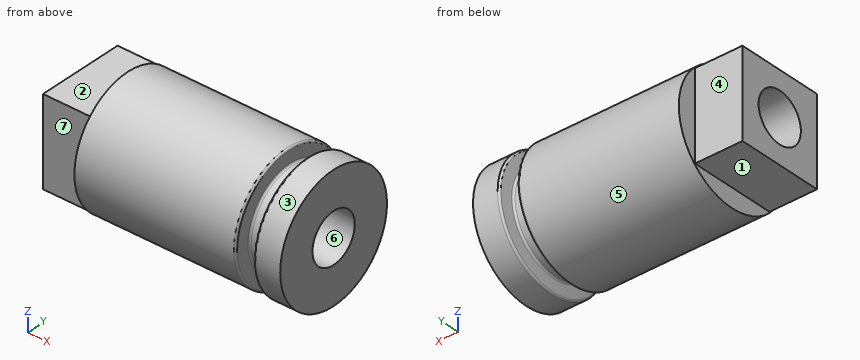
from build123d import *

# Parameters (mm, degrees)
F2_W     = 17.4498
F2_H     = 17.4498
F3_DEPTH = 9.525
F4_R     = 4.953
F5_DEPTH = 50.801


with BuildPart() as f1:
    # F0 (on Front) → F1 (revolve)
    with BuildSketch(Plane.XZ):
        with BuildLine():
            Line((11.316179, 12.4968), (-20.6375, 12.4968))
            Line((-20.6375, 12.4968), (-20.6375, 0))
            Line((-20.6375, 0), (20.6375, 0))
            Line((20.6375, 0), (20.6375, 12.4968))
            Line((20.6375, 12.4968), (15.709421, 12.4968))
            ThreePointArc((15.709421, 12.4968), (15.452021, 12.396703), (15.329871, 12.149006))
            Line((15.329871, 12.149006), (15.130728, 9.872794))
            ThreePointArc((15.130728, 9.872794), (15.008578, 9.625097), (14.751178, 9.525))
            Line((14.751178, 9.525), (12.274422, 9.525))
            ThreePointArc((12.274422, 9.525), (12.017022, 9.625097), (11.894872, 9.872794))
            Line((11.894872, 9.872794), (11.695729, 12.149006))
            ThreePointArc((11.695729, 12.149006), (11.573579, 12.396703), (11.316179, 12.4968))
        make_face()
    revolve(axis=Axis((-2.210241, 0, 0), (-1, 0, 0)))

    # F2 (on face) → F3 (join)
    with BuildSketch(Plane(origin=(-20.6375, 0, 0), x_dir=(0, -1, 0), z_dir=(-1, 0, 0))):
        Rectangle(F2_W, F2_H)
    extrude(amount=F3_DEPTH)

    # F4 (on face) → F5 (cut, through all)
    with BuildSketch(Plane.YZ.offset(20.6375)):
        Circle(F4_R)
    extrude(amount=-F5_DEPTH, mode=Mode.SUBTRACT)


solid = f1.part
For this review, take the finished solid that the model builds, in its own axes (mm). Face numbers are marked on the shaded views. A direction names the side the tool comes from. Give positions to 0.01 mm unless a question says otherwise; leave off trailing zeros. Order: outer loops, then holes, each group sorted by start corner. A loop starts at its lowest first (then second) coordinate and runs counter-clockwise, first axis right, second up. Notation, with made-up numbers: (63, 17) - (84, 17) arc R10 ccw to (84, 34) - close; hole circle Ø2 at (42, -11). An arc over 180 degrees is marked (long way). Answer as a JSON object with one key per item and string values. Group by question number.
Item 1: Machinability: for the marked faces 1, 2, 3 and 4, which of the approach directions +Z, -Z, +X, -X, +Y, -Y give a long, thin tool a straight path to every point of the face, cutting with its end or side? Answer none if there is none.
Item 2: Draft analysis for pull direction Z (two halves, no side actions). For the marked faces 5, 6 and 7, state which applies: pulls with the +Z half, pulls with the -Z half, needs draft (parallel to the pull), parting line crosses it, or undercut.
Item 3: Clearance check with flat-ended pins moving along their axes: pin 1 Ø1.5 at (x, y) = (-11.5, -7) entering from -Z; pin 2 Ø5 at (x, z) = (-25, 0) entering from -Y; pin 3 Ø5 at (x, y) = (-3, 7) entering from -Z. State where each tip first meets the part, or that it passes through.
Item 4: Take a section at A-A on z = 0. Give the boundary of the cut face in (x, y) (1 decimal), and give its area (3 significant figures).
Item 5: Take a section at D-D on x = -9. Give the boundary of the cut face in (y, z).
Item 6: Take a section at C-C on x = -25.5. Give the boundary of the cut face in (y, z), and give its area (3 significant figures).
Item 7: Wall thickness on line 1 along X through (y, z) = (10.5, 6) (1 decimal); line 2 along Z through (x, y) = (-18, 2.5); line 3 along Z through (x, y) = (-1.5, 4.25): over which ranges is each line inside the solid? List them lowest first.
Reported:
{
 "1": {"face 1": "-Z, -X, +Y, -Y", "face 2": "+Z, -X, +Y, -Y", "face 3": "+X, -X", "face 4": "+Z, -Z, -X, +Y"},
 "2": {"face 5": "parting line crosses it", "face 6": "undercut", "face 7": "needs draft"},
 "3": {"pin 1": "z = -10.82", "pin 2": "y = -8.72", "pin 3": "z = -11.66"},
 "4": {"outline": "(-30.2, -8.7) - (-20.6, -8.7) - (-20.6, -12.5) - (11.3, -12.5) arc R0.4 ccw to (11.7, -12.1) - (11.9, -9.9) arc R0.4 cw to (12.3, -9.5) - (14.8, -9.5) arc R0.4 cw to (15.1, -9.9) - (15.3, -12.1) arc R0.4 ccw to (15.7, -12.5) - (20.6, -12.5) - (20.6, -5) - (-30.2, -5) - close; (-30.2, 5) - (20.6, 5) - (20.6, 12.5) - (15.7, 12.5) arc R0.4 ccw to (15.3, 12.1) - (15.1, 9.9) arc R0.4 cw to (14.8, 9.5) - (12.3, 9.5) arc R0.4 cw to (11.9, 9.9) - (11.7, 12.1) arc R0.4 ccw to (11.3, 12.5) - (-20.6, 12.5) - (-20.6, 8.7) - (-30.2, 8.7) - close", "area": "674 mm^2"},
 "5": {"outline": "circle Ø24.99 at (0, 0); hole circle Ø9.91 at (0, 0)"},
 "6": {"outline": "(-8.72, -8.72) - (8.72, -8.72) - (8.72, 8.72) - (-8.72, 8.72) - close; hole circle Ø9.91 at (0, 0)", "area": "227 mm^2"},
 "7": {"line 1": "-20.6 to 11.7, 15.3 to 20.6", "line 2": "-12.24 to -4.28, 4.28 to 12.24", "line 3": "-11.75 to -2.54, 2.54 to 11.75"}
}
